```python
from build123d import *

# Parameters (mm, degrees)
SKETCH1_R               = 7
BOSS_EXTRUDE1_DEPTH     = 44
SKETCH1_2_R             = 7
BOSS_EXTRUDE2_DEPTH     = 44
CUT_EXTRUDE1_DEPTH      = 1
CUT_EXTRUDE1_DEPTH_BACK = 19
SKETCH4_W               = 50.710370583
SKETCH4_H               = 19
CUT_EXTRUDE2_DEPTH      = 52
SKETCH5_R               = 5.5
CUT_EXTRUDE3_DEPTH      = 45
CUT_EXTRUDE4_DEPTH      = 24
CUT_EXTRUDE12_DEPTH     = 7
CUT_EXTRUDE13_DEPTH     = 25


with BuildPart() as part:
    # Sketch1 → Boss-Extrude1 (new body)
    with BuildSketch(Plane.XY):
        with BuildLine():
            Line((-7, -14), (25.575538911, -14))
            ThreePointArc((25.575538911, -14), (28.840774692, -15.213413768), (30.521177653, -18.264705882))
            ThreePointArc((30.521177653, -18.264705882), (32.858007856, -26.115672061), (37.296980053, -33))
            Line((37.296980053, -33), (43, -33))
            Line((43, -33), (72, 1))
            Line((72, 1), (72, 20))
            Line((72, 20), (67, 25))
            Line((67, 25), (43, 25))
            ThreePointArc((43, 25), (34.561098706, 15.982044142), (22.361380836, 14.057085233))
            Line((22.361380836, 14.057085233), (0, 18))
            Line((0, 18), (-7, 18))
            Line((-7, 18), (-14, 11))
            Line((-14, 11), (-14, -7))
            Line((-14, -7), (-7, -14))
        make_face()
        Circle(SKETCH1_R, mode=Mode.SUBTRACT)
    extrude(amount=BOSS_EXTRUDE1_DEPTH)

    # Sketch1_2 → Boss-Extrude2 (add)
    with BuildSketch(Plane.XY):
        with BuildLine():
            Line((-7, -14), (25.575538911, -14))
            ThreePointArc((25.575538911, -14), (28.840774692, -15.213413768), (30.521177653, -18.264705882))
            ThreePointArc((30.521177653, -18.264705882), (32.858007856, -26.115672061), (37.296980053, -33))
            Line((37.296980053, -33), (43, -33))
            Line((43, -33), (72, 1))
            Line((72, 1), (72, 20))
            Line((72, 20), (67, 25))
            Line((67, 25), (43, 25))
            ThreePointArc((43, 25), (34.561098706, 15.982044142), (22.361380836, 14.057085233))
            Line((22.361380836, 14.057085233), (0, 18))
            Line((0, 18), (-7, 18))
            Line((-7, 18), (-14, 11))
            Line((-14, 11), (-14, -7))
            Line((-14, -7), (-7, -14))
        make_face()
        Circle(SKETCH1_2_R, mode=Mode.SUBTRACT)
    extrude(amount=BOSS_EXTRUDE2_DEPTH)

    # Sketch3 → Cut-Extrude1 (cut, two sides)
    with BuildSketch(Plane.XY.offset(44)) as cut_extrude1_sk:
        Polygon((-150.317212119, -14), (25.575538911, -14), (59.205882353, -14), (235.098633383, -14), (235.098633383, -365.78550206), (-150.317212119, -365.78550206), align=None)
    extrude(amount=CUT_EXTRUDE1_DEPTH, mode=Mode.SUBTRACT)
    extrude(cut_extrude1_sk.sketch, amount=-CUT_EXTRUDE1_DEPTH_BACK, mode=Mode.SUBTRACT)

    # Sketch4 → Cut-Extrude2 (cut, through all)
    with BuildSketch(Plane(origin=(0, 18, 0), x_dir=(1, 0, 0), z_dir=(0, 1, 0))):
        with Locations((-5.355185292, -34.5)):
            Rectangle(SKETCH4_W, SKETCH4_H)
    extrude(amount=-CUT_EXTRUDE2_DEPTH, mode=Mode.SUBTRACT)

    # Sketch5 → Cut-Extrude3 (cut, through all)
    with BuildSketch(Plane.XY.offset(44)):
        with Locations((58, 11)):
            Circle(SKETCH5_R)
    extrude(amount=-CUT_EXTRUDE3_DEPTH, mode=Mode.SUBTRACT)

    # Sketch9 → Cut-Extrude4 (cut)
    with BuildSketch(Plane(origin=(0, 0, 12), x_dir=(-1, 0, 0), z_dir=(0, 0, -1))):
        with BuildLine():
            Line((-72, 20), (-67, 25))
            Line((-67, 25), (-43, 25))
            ThreePointArc((-43, 25), (-39.021244343, 19.259333621), (-33.236936549, 15.344294617))
            ThreePointArc((-33.236936549, 15.344294617), (-44.184262982, -1.419294771), (-61.764705882, -11))
            Line((-61.764705882, -11), (-72, 1))
            Line((-72, 1), (-72, 20))
        make_face()
    extrude(amount=-CUT_EXTRUDE4_DEPTH, mode=Mode.SUBTRACT)

    # Sketch16 → Cut-Extrude12 (cut)
    with BuildSketch(Plane.XY.offset(44)):
        with BuildLine():
            Line((21, 13.281706793), (21, -13))
            Line((21, -13), (58.744476296, -13))
            Line((58.744476296, -13), (71, 1.368545033))
            Line((71, 1.368545033), (71, 19.585786438))
            Line((71, 19.585786438), (66.585786438, 24))
            Line((66.585786438, 24), (43.636084685, 24))
            ThreePointArc((43.636084685, 24), (34.740005768, 14.948047079), (22.187732658, 13.07227748))
            Line((22.187732658, 13.07227748), (21, 13.281706793))
        make_face()
    extrude(amount=-CUT_EXTRUDE12_DEPTH, mode=Mode.SUBTRACT)

    # Sketch17 → Cut-Extrude13 (cut)
    with BuildSketch(Plane.XY.offset(37)):
        with BuildLine():
            Line((58.744476296, -13), (59.986847747, -11.543426575))
            ThreePointArc((59.986847747, -11.543426575), (43.310181683, -1.972127362), (32.646682943, 14.028208705))
            ThreePointArc((32.646682943, 14.028208705), (27.481076416, 12.851449437), (22.187732658, 13.07227748))
            Line((22.187732658, 13.07227748), (21, 13.281706793))
            Line((21, 13.281706793), (21, -13))
            Line((21, -13), (58.744476296, -13))
        make_face()
    extrude(amount=-CUT_EXTRUDE13_DEPTH, mode=Mode.SUBTRACT)


solid = part.part
```
Verification items for the finished model (mm, model axes). A direction names the side the tool comes from. Coordinates: 2 decimals unless noted, no trailing zeros. Order: outer loops, then holes, each group sorted by start corner. A loop starts at its lowest first (then second) coordinate and runs counter-clockwise, first axis right, second up. Notation, with made-up numbers: (32, 50.5) - (51, 50.5) arc R32 ccw to (51, 88.5) - close; hole circle Ø7 at (-25.75, 63.25). An arc over 180 degrees is marked (long way). Return JSON: item names as keys, results as strings.
(1) Section check A-A, the plane y = 21. Record the cut outline in (x, z), and give its area (3 significant figures).
Filled sheet:
{"outline": "(40.58, 0) - (71, 0) - (71, 12) - (40.58, 12) - close; (40.58, 36) - (71, 36) - (71, 44) - (69.59, 44) - (69.59, 37) - (41.83, 37) - (41.83, 44) - (40.58, 44) - close", "area": "414 mm^2"}
(2) Section check D-D, the plane y = 0. Record the cut outline in (x, z), and give its area (3 significant figures).
Filled sheet:
{"outline": "(-14, 0) - (-7, 0) - (-7, 25) - (-14, 25) - close; (7, 0) - (71.15, 0) - (71.15, 12) - (42.72, 12) - (42.72, 36) - (71.15, 36) - (71.15, 44) - (69.83, 44) - (69.83, 37) - (41.34, 37) - (41.34, 12) - (21, 12) - (21, 44) - (20, 44) - (20, 25) - (7, 25) - close", "area": "1,220 mm^2"}
(3) Section check B-B, the plane z = 22. Record the cut outline in (x, y).
Filled sheet:
{"outline": "(-14, -7) - (-7, -14) - (25.58, -14) arc R5 cw to (30.52, -18.26) arc R29 ccw to (37.3, -33) - (43, -33) - (61.76, -11) arc R41 cw to (33.24, 15.34) arc R19 cw to (22.36, 14.06) - (0, 18) - (-7, 18) - (-14, 11) - close; hole circle Ø14 at (0, 0); hole (21, -13) - (58.74, -13) - (59.99, -11.54) arc R42 cw to (32.65, 14.03) arc R20 cw to (22.19, 13.07) - (21, 13.28) - close"}
(4) Mould release check, pull along X, two halves, no side actions. Record for faces 4 (the flat face through (55, 25, 40)), 5 (the flat face through (11.34, 16, 11.91)), 6 (the flat face through (70, 22, 40)): pulls with the +X half, pulls with the -X half, needs draft (parallel to the pull), parting line crosses it, or undercut.
Filled sheet:
{"face 4": "needs draft", "face 5": "undercut", "face 6": "pulls with the +X half"}
(5) Thickness scan on line 1 along Z through (x, y) = (46.5, 4); line 2 along X through (y, z) = (1.5, 24); line 3 along Y through (x, z) = (53.5, 39.5). Record the ranges inside material, lowest first.
Filled sheet:
{"line 1": "z = 0 to 12, 36 to 37", "line 2": "x = -14 to -6.84, 6.84 to 21, 40 to 41.32", "line 3": "y = -14 to -13, 24 to 25"}
(6) Access from +Z, -Z, +X, -X, +Y, -Y to the whole of each face (thin tool, end or side, straight path). Record for faces 1 (the flat face through (26, -14, 27)), 2 (the flat face through (52, 11, 36)), 3 (the flat face through (21, 0, 28)).
Filled sheet:
{"face 1": "+Z, -X, -Y", "face 2": "+X, +Y", "face 3": "+Z"}
(7) Section check C-C, the plane x = 23.5. Record the cut outline in (y, z), and give its area (3 significant figures).
Filled sheet:
{"outline": "(-14, 0) - (13.89, 0) - (13.89, 44) - (12.89, 44) - (12.89, 12) - (-13, 12) - (-13, 44) - (-14, 44) - close", "area": "399 mm^2"}
(8) Go/stop test with flat-tipped pins: pin 1 (11 mm diameter, centred on x = 62, y = -0.5, fed in from -Z); pin 2 (7.5 mm diameter, centred on x = -3.5, z = 10, fed in from +Y); pin 3 (18 mm diameter, centred on x = 57, y = 14.5, fed in from +Z); pin 4 (13 mm diameter, centred on y = 4, z = 22.5, fed in from +X). Record where each tip stops, or that it passes through.
Filled sheet:
{"pin 1": "stops at z = 0", "pin 2": "stops at y = 18", "pin 3": "stops at z = 37", "pin 4": "stops at x = 45.4"}
